```python
from build123d import *

# Parameters (mm, degrees)
BOSS_EXTRU_1_DEPTH      = 6
ESQUISSE2_R             = 1.5
ESQUISSE2_R_2           = 1.25
ENL_V_MAT_EXTRU_1_DEPTH = 6


with BuildPart() as part:
    # Esquisse1 → Boss.-Extru.1 (new body)
    with BuildSketch(Plane.XY):
        with BuildLine():
            Line((-31, 1.5), (-31, 7.5))
            Line((-31, 7.5), (31, 7.5))
            Line((31, 7.5), (31, 1.5))
            Line((31, 1.5), (30.809475019, 1.5))
            ThreePointArc((30.809475019, 1.5), (25, 6), (19.190524981, 1.5))
            Line((19.190524981, 1.5), (-19.190524981, 1.5))
            ThreePointArc((-19.190524981, 1.5), (-25, 6), (-30.809475019, 1.5))
            Line((-30.809475019, 1.5), (-31, 1.5))
        make_face()
    extrude(amount=BOSS_EXTRU_1_DEPTH)

    # Esquisse2 → Enlèv. mat.-Extru.1 (cut)
    with BuildSketch(Plane(origin=(0, 7.5, 0), x_dir=(1, 0, 0), z_dir=(0, 1, 0))):
        with Locations(Location((-16, -3, 0), (0, 0, 270))):
            Circle(ESQUISSE2_R)
        with Locations(Location((16, -3, 0), (0, 0, 270))):
            Circle(ESQUISSE2_R)
        with Locations(Location((0, -3, 0), (0, 0, 270))):
            Circle(ESQUISSE2_R_2)
    extrude(amount=-ENL_V_MAT_EXTRU_1_DEPTH, mode=Mode.SUBTRACT)


solid = part.part
```
Build history of the part. All positions in model axes, mm. Coordinates: 2 decimals unless noted, no trailing zeros. Order: outer loops, then holes, each group sorted by start corner. A loop starts at its lowest first (then second) coordinate and runs counter-clockwise, first axis right, second up.
Item 1: Drill centre lines: L1, parallel to X at y = 3.2, z = 1.1; L2, parallel to X at y = 3.65, z = 3; L3, parallel to X at y = 3.9, z = 3. Where is each one in solid material? Low to high.
Filled in:
L1: x = -31 to -30.08, -19.92 to 19.92, 30.08 to 31
L2: x = -31 to -29.76, -20.24 to -17.5, -14.5 to -1.25, 1.25 to 14.5, 17.5 to 20.24, 29.76 to 31
L3: x = -31 to -29.56, -20.44 to -17.5, -14.5 to -1.25, 1.25 to 14.5, 17.5 to 20.44, 29.56 to 31
Item 2: Saw through at C-C on z = 3. List the corners of the cut face in (x, y).
Filled in:
outline: (-31, 1.5) - (-30.81, 1.5) arc R6 cw to (-19.19, 1.5) - (-17.5, 1.5) - (-17.5, 7.5) - (-31, 7.5) - close; (-14.5, 1.5) - (-1.25, 1.5) - (-1.25, 7.5) - (-14.5, 7.5) - close; (1.25, 1.5) - (14.5, 1.5) - (14.5, 7.5) - (1.25, 7.5) - close; (17.5, 1.5) - (19.19, 1.5) arc R6 cw to (30.81, 1.5) - (31, 1.5) - (31, 7.5) - (17.5, 7.5) - close
Item 3: Saw through at A-A on y = 6.65. List the corners of the cut face in (x, z), then the cut area to 3 significant figures.
Filled in:
outline: (-31, 0) - (31, 0) - (31, 6) - (-31, 6) - close; hole circle Ø3 at (-16, 3); hole circle Ø2.5 at (0, 3); hole circle Ø3 at (16, 3)
area: 353 mm2
Item 4: Mould opens along X. For faces 1 (the flat face through (0, 5, 6)), 2 (the cylindrical face through (25, 6, 3)), 3 (the flat face through (31, 5, 3)) say: released by +X, released by -X, zero draft, split by the parting line, or undercut.
Filled in:
face 1: zero draft
face 2: undercut
face 3: released by +X
Item 5: Saw through at B-B on x = 0. List the corners of the cut face in (y, z), then the cut area to 3 significant figures.
Filled in:
outline: (1.5, 0) - (7.5, 0) - (7.5, 1.75) - (1.5, 1.75) - close; (1.5, 4.25) - (7.5, 4.25) - (7.5, 6) - (1.5, 6) - close
area: 21.0 mm2
Item 6: Drop flat-ended pins along their axis: pin 1 Ø1.5 at (x, y) = (-19, 2) entering from -Z; pin 2 Ø1.8 at (x, z) = (16, 3) entering from +Y. Give the stop position or say it passes through.
Filled in:
pin 1: stops at z = 0
pin 2: passes through
Item 7: Saw through at D-D on y = 2.95. List the corners of the cut face in (x, z).
Filled in:
outline: (-31, 0) - (-30.22, 0) - (-30.22, 6) - (-31, 6) - close; (-19.78, 0) - (19.78, 0) - (19.78, 6) - (-19.78, 6) - close; (30.22, 0) - (31, 0) - (31, 6) - (30.22, 6) - close; hole circle Ø3 at (-16, 3); hole circle Ø2.5 at (0, 3); hole circle Ø3 at (16, 3)
